Model file for the job. Use its own axes, mm. Face numbers are marked on the shaded views. Coordinates: 2 decimals unless noted, no trailing zeros. Write each loop counter-clockwise with the first axis right and the second up, starting at its lowest first coordinate (ties: lowest second). Pieces come first, ordered by that corner, then holes.
Q1. Pull direction X, two halves, no side cores. Call the marked faces 1, 2, 3 and 4: released by +X, released by -X, zero draft, split by the parting line, or undercut.
Q2. Band-saw the part on D-D, the plane y = 5. Write the cut outline in (x, z), plus the area to 3 significant figures.
Q3. Band-saw the part on C-C, the plane x = -0.25. Write the cut outline in (y, z), plus the area to 3 significant figures.
Q4. Drill centre lines: probe 1 along X at (y, z) = (6.25, 0); probe 2 along Y at (x, z) = (-1.75, -5.75); probe 3 along X at (y, z) = (3.25, -0.5). Where is each one in solid material? Low to high.
Q5. Pin check, flat tips, straight feed: P1, Ø3, axis at x = -5.5, z = -4.5, coming from the -Y side; P2, Ø4, axis at x = -6, z = -4, coming from the +Y side; P3, Ø5, axis at y = 14.5, z = 2.5, coming from the -X side; P4, Ø1.5, axis at x = -2.5, y = 8.5, coming from the +Z side. Stop position of each tip, or through.
Q6. Band-saw the part on B-B, the plane z = 0. Write the cut outline in (x, y).
Q7. Band-saw the part on A-A, the plane x = -2. Write the cut outline in (y, z), plus the area to 3 significant figures.
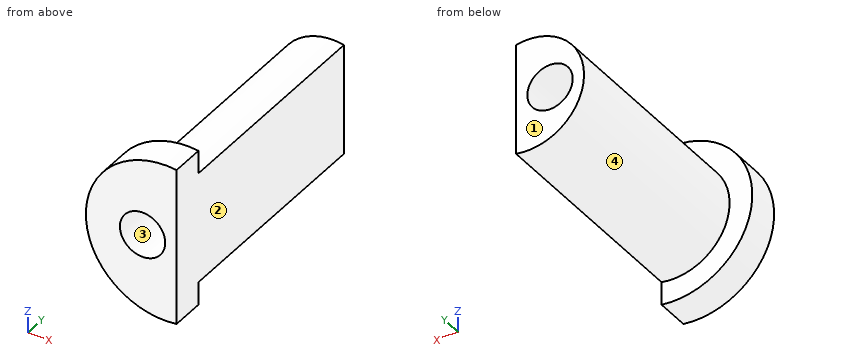
from build123d import *

# Parameters (mm, degrees)
SKETCH_1_R          = 7
EXTRUDE_1_DEPTH     = 3
SKETCH_2_R          = 5
EXTRUDE_2_DEPTH     = 20
SKETCH_3_R          = 2
CUT_EXTRUDE_1_DEPTH = 26.039968051
SKETCH_4_W          = 8.616079813
SKETCH_4_H          = 14.040723598
CUT_EXTRUDE_2_DEPTH = 26.039968051


with BuildPart() as part:
    # 草图1 → 凸台-拉伸1 (new body)
    with BuildSketch(Plane(origin=(0, 0, 0), x_dir=(1, 0, 0), z_dir=(0, 1, 0))):
        with Locations(Location((0, 0, 0), (0, 0, 270))):
            Circle(SKETCH_1_R)
    extrude(amount=EXTRUDE_1_DEPTH)

    # 草图2 → 凸台-拉伸2 (add)
    with BuildSketch(Plane(origin=(0, 3, 0), x_dir=(1, 0, 0), z_dir=(0, 1, 0))):
        with Locations(Location((0, 0, 0), (0, 0, 270))):
            Circle(SKETCH_2_R)
    extrude(amount=EXTRUDE_2_DEPTH)

    # 草图3 → 切除-拉伸1 (cut, through all)
    with BuildSketch(Plane(origin=(0, 23, 0), x_dir=(1, 0, 0), z_dir=(0, 1, 0))):
        with Locations(Location((-2, 0, 0), (0, 0, 270))):
            Circle(SKETCH_3_R)
    extrude(amount=-CUT_EXTRUDE_1_DEPTH, mode=Mode.SUBTRACT)

    # 草图4 → 切除-拉伸2 (cut, through all)
    with BuildSketch(Plane(origin=(0, 23, 0), x_dir=(1, 0, 0), z_dir=(0, 1, 0))):
        with Locations((5.308039907, -0.092158569)):
            Rectangle(SKETCH_4_W, SKETCH_4_H)
    extrude(amount=-CUT_EXTRUDE_2_DEPTH, mode=Mode.SUBTRACT)


solid = part.part
Answer sheet:
1. face 1: zero draft
1. face 2: released by +X
1. face 3: undercut
1. face 4: split by the parting line
2. outline: (1, -4.9) - (1, 4.9) arc R5 ccw (long way) to start; hole circle Ø4 at (-2, 0)
2. area: 36.6 mm2
3. outline: (0, -7) - (3, -7) - (3, -4.99) - (23, -4.99) - (23, -0.97) - (0, -0.97) - close; (0, 0.97) - (23, 0.97) - (23, 4.99) - (3, 4.99) - (3, 7) - (0, 7) - close
3. area: 197 mm2
4. probe 1: x = -5 to -4, 0 to 1
4. probe 2: y = 0 to 3
4. probe 3: x = -4.97 to -3.94, -0.06 to 1
5. P1: stops at y = 0
5. P2: stops at y = 3
5. P3: stops at x = -5
5. P4: stops at z = 4.68
6. outline: (-7, 0) - (-4, 0) - (-4, 23) - (-5, 23) - (-5, 3) - (-7, 3) - close; (0, 0) - (1, 0) - (1, 23) - (0, 23) - close
7. outline: (0, -6.71) - (3, -6.71) - (3, -4.58) - (23, -4.58) - (23, -2) - (0, -2) - close; (0, 2) - (23, 2) - (23, 4.58) - (3, 4.58) - (3, 6.71) - (0, 6.71) - close
7. area: 132 mm2
